CAD build for the part. Positions are in the model's coordinates, mm. Face numbers are marked on the shaded views. A direction names the side the tool comes from. Coordinates: 2 decimals unless noted, no trailing zeros. Write each loop counter-clockwise with the first axis right and the second up, starting at its lowest first coordinate (ties: lowest second). Pieces come first, ordered by that corner, then holes. Notation, with made-up numbers: (-4.5, 76) -> (24.5, 76) arc R25 cw to (24.5, 96) -> close; hole circle Ø8 at (82, 8.5). An arc over 180 degrees is marked (long way). Answer as CSV lines item,"result".
```python
from build123d import *

# Parameters (mm, degrees)
F1_DEPTH = 12.5
F2_R     = 5


# Not quite as in the source:
# - a feature names something its author has since deleted; it is built from what else it names


with BuildPart() as f1:
    # F0 (on Front) → F1 (new body, symmetric)
    with BuildSketch(Plane.XZ):
        Polygon((-49.1098842621, 66.8063223362), (-53.1098842621, 66.8063223362), (-53.1098842621, -33.1936776638), (46.8901157379, -33.1936776638), (46.8901157379, 66.8063223362), (42.8901157379, 66.8063223362), (42.8901157379, -29.1936776638), (-49.1098842621, -29.1936776638), align=None)
    extrude(amount=F1_DEPTH, both=True)

    # F2
    f2_edges = [f1.edges().sort_by_distance(p)[0] for p in [
        (-51.109884, -12.5, 66.806322),
        (-51.109884, 12.5, 66.806322),
        (44.890116, -12.5, 66.806322),
        (44.890116, 12.5, 66.806322),
        (46.890116, 0, -33.193678),
        (-53.109884, 0, -33.193678),
    ]]
    fillet(f2_edges, radius=F2_R)


solid = f1.part
```
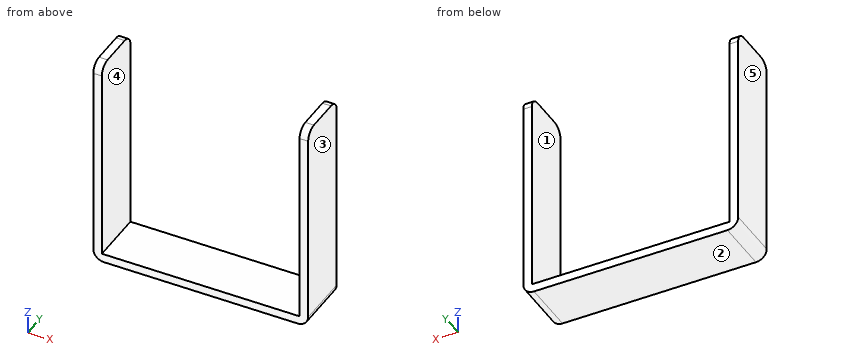
Item 1: Saw through at B-B on y = -0.5. Give the cut face in (x, z), and give its area (3 significant figures).
Answer below:
outline,"(-53.11, -28.19) arc R5 ccw to (-48.11, -33.19) -> (41.89, -33.19) arc R5 ccw to (46.89, -28.19) -> (46.89, 66.81) -> (42.89, 66.81) -> (42.89, -29.19) -> (-49.11, -29.19) -> (-49.11, 66.81) -> (-53.11, 66.81) -> close"
area,"1,160 mm2"
Item 2: 3-axis set-ups, long thin cutter, end or side, ignore diameter. For the marked faces 4 and 5: which of +Z, -Z, +X, -X, +Y, -Y reach the whole face in a straight line?
Answer below:
face 4,"+Z, +Y, -Y"
face 5,"+Z, -Z, -X, +Y, -Y"
Item 3: Saw through at A-A on z = 39.5. Give the cut face in (x, y).
Answer below:
outline,"(-53.11, -12.5) -> (-49.11, -12.5) -> (-49.11, 12.5) -> (-53.11, 12.5) -> close; (42.89, -12.5) -> (46.89, -12.5) -> (46.89, 12.5) -> (42.89, 12.5) -> close"
Item 4: Two-plate mould, pull along X, no slides. Class the marked faces 1, 2 and 3: pulls with the +X half, pulls with the -X half, needs draft (parallel to the pull), parting line crosses it, or undercut.
Answer below:
face 1,"undercut"
face 2,"needs draft"
face 3,"pulls with the +X half"
Item 5: Wall check: line 1 (X direction, y = -4, z = 18); line 2 (Z direction, x = -28.5, y = -3.5). Give the ranges that are in metal, low to high. Write a range as from..to.
Answer below:
line 1,"x = -53.11..-49.11, 42.89..46.89"
line 2,"z = -33.19..-29.19"
Item 6: Flat gauge pin, fed straight in: pin 1 (3 mm diameter, centred on x = -32.5, y = -3, fed in from +Z). Where does the tip first touch, or does it go through?
Answer below:
pin 1,"stops at z = -29.19"
Item 7: Saw through at C-C on x = 25.5. Give the cut face in (y, z), and give its area (3 significant figures).
Answer below:
outline,"(-12.5, -33.19) -> (12.5, -33.19) -> (12.5, -29.19) -> (-12.5, -29.19) -> close"
area,"100 mm2"
Item 8: Saw through at D-D on y = -11. Give the cut face in (x, z), and give its area (3 significant figures).
Answer below:
outline,"(-53.11, -28.19) arc R5 ccw to (-48.11, -33.19) -> (41.89, -33.19) arc R5 ccw to (46.89, -28.19) -> (46.89, 65.38) -> (42.89, 65.38) -> (42.89, -29.19) -> (-49.11, -29.19) -> (-49.11, 65.38) -> (-53.11, 65.38) -> close"
area,"1,150 mm2"
